from build123d import *

# Parameters (mm, degrees)
SKETCH1_R           = 19.24
BOSS_EXTRUDE1_DEPTH = 1.5
SKETCH2_R           = 3.5
SKETCH2_R_2         = 2
BOSS_EXTRUDE2_DEPTH = 15
FILLET1_R           = 1


with BuildPart() as part:
    # Sketch1 → Boss-Extrude1 (new body)
    with BuildSketch(Plane(origin=(0, 0, 0), x_dir=(1, 0, 0), z_dir=(0, 1, 0))):
        with Locations(Location((0, 0, 0), (0, 0, 270))):
            Circle(SKETCH1_R)
        with BuildLine():
            Line((14.66, 1.27), (12.12, 1.27))
            ThreePointArc((12.12, 1.27), (10.85, 0), (12.12, -1.27))
            Line((12.12, -1.27), (14.66, -1.27))
            ThreePointArc((14.66, -1.27), (15.93, 0), (14.66, 1.27))
        make_face(mode=Mode.SUBTRACT)
        with BuildLine():
            Line((-14.66, -1.27), (-12.12, -1.27))
            ThreePointArc((-12.12, -1.27), (-10.85, 0), (-12.12, 1.27))
            Line((-12.12, 1.27), (-14.66, 1.27))
            ThreePointArc((-14.66, 1.27), (-15.93, 0), (-14.66, -1.27))
        make_face(mode=Mode.SUBTRACT)
    extrude(amount=BOSS_EXTRUDE1_DEPTH)

    # Sketch2 → Boss-Extrude2 (add)
    with BuildSketch(Plane(origin=(0, 0, 0), x_dir=(-1, 0, 0), z_dir=(0, -1, 0))):
        with Locations(Location((0, 0, 0), (0, 0, 270))):
            Circle(SKETCH2_R)
        with Locations(Location((0, 0, 0), (0, 0, 90))):
            Circle(SKETCH2_R_2, mode=Mode.SUBTRACT)
    extrude(amount=BOSS_EXTRUDE2_DEPTH)

    # Fillet1
    fillet1_edges = [part.edges().sort_by_distance(p)[0] for p in [
        (0, 0, -3.5),
    ]]
    fillet(fillet1_edges, radius=FILLET1_R)


solid = part.part
Source: CAD feature listing. Evaluate the final solid. Frame: model axes, mm. A direction names the side the tool comes from. Give positions to 0.01 mm unless a question says otherwise; leave off trailing zeros. Write each loop counter-clockwise with the first axis right and the second up, starting at its lowest first coordinate (ties: lowest second). Pieces come first, ordered by that corner, then holes. Notation, with made-up numbers: (78.5, 25) -> (122.5, 25) arc R29 cw to (122.5, 49) -> close; hole circle Ø3 at (28, 66.5). An arc over 180 degrees is marked (long way). Return JSON: item names as keys, results as strings. Group by question number.
1. Section A-A, the plane z = 0. Output: boundary loops of the cut face in (x, y), then the cut area to 3 significant figures.
2. Mould query, pull axis X, two halves, no side actions, for faces 1 (the face through (3.417, -7.902, -0.759)), 2 (the face through (0, 1.5, 0)), 3 (the face through (-2, -7, 0)), 4 (the face through (-15.93, 0.74, -0.03)). Classes: +X half, -X half, draft (parallel to the pull), parting line (faces both ways), or undercut.
3. Section D-D, the plane z = -14. Output: boundary loops of the cut face in (x, y), then the cut area to 3 significant figures.
4. Section B-B, the plane y = -14. Output: boundary loops of the cut face in (x, z), then the cut area to 3 significant figures.
5. Section C-C, the plane x = -9. Output: boundary loops of the cut face in (y, z), then the cut area to 3 significant figures.
6. Material intervals for line 1 (X direction, y = -3.5, z = 0); line 2 (Y direction, x = -6, z = -6); line 3 (Z direction, x = -1, y = -13.5), sorted ascending. Write a range as from..to.
7. Pin query (flat end, axial travel): pin 1 Ø1.6 at (x, y) = (13, 1) entering from +Z; pin 2 Ø3 at (x, y) = (-2.5, -3.5) entering from +Z; pin 3 Ø0.8 at (x, y) = (-14, 0.5) entering from -Z; pin 4 Ø19 at (x, z) = (-7, -6) entering from -Y. Return the tip coordinate at first contact, or that it passes through.
8. Access query for faces 5 (the face through (-13, 1, -1.27)), 6 (the face through (0, 0, 0)), 7 (the face through (2, -15, 2)). Directions: +Z, -Z, +X, -X, +Y, -Y. A direction counts if a zero-diameter tool reaches every point of the face in a straight line with its end or side. Return the directions, or none.
Determined:
{
 "1": {"outline": "(-19.24, 0) -> (-15.93, 0) -> (-15.93, 1.5) -> (-19.24, 1.5) -> close; (-10.85, 0) -> (-4.5, 0) arc R1 cw to (-3.5, -1) -> (-3.5, -15) -> (-2, -15) -> (-2, 0) -> (2, 0) -> (2, -15) -> (3.5, -15) -> (3.5, -1) arc R1 cw to (4.5, 0) -> (10.85, 0) -> (10.85, 1.5) -> (-10.85, 1.5) -> close; (15.93, 0) -> (19.24, 0) -> (19.24, 1.5) -> (15.93, 1.5) -> close", "area": "87.9 mm2"},
 "2": {"face 1": "parting line", "face 2": "draft", "face 3": "undercut", "face 4": "undercut"},
 "3": {"outline": "(-13.2, 0) -> (13.2, 0) -> (13.2, 1.5) -> (-13.2, 1.5) -> close", "area": "39.6 mm2"},
 "4": {"outline": "circle Ø7 at (0, 0); hole circle Ø4 at (0, 0)", "area": "25.9 mm2"},
 "5": {"outline": "(0, -17.01) -> (1.5, -17.01) -> (1.5, 17.01) -> (0, 17.01) -> close", "area": "51.0 mm2"},
 "6": {"line 1": "x = -3.5..-2, 2..3.5", "line 2": "y = 0..1.5", "line 3": "z = -3.35..-1.73, 1.73..3.35"},
 "7": {"pin 1": "stops at z = 14.88", "pin 2": "stops at z = 3.35", "pin 3": "stops at z = -13.61", "pin 4": "stops at y = -15"},
 "8": {"face 5": "+Y, -Y", "face 6": "-Y", "face 7": "+Z, -Z, +X, -X, -Y"}
}
